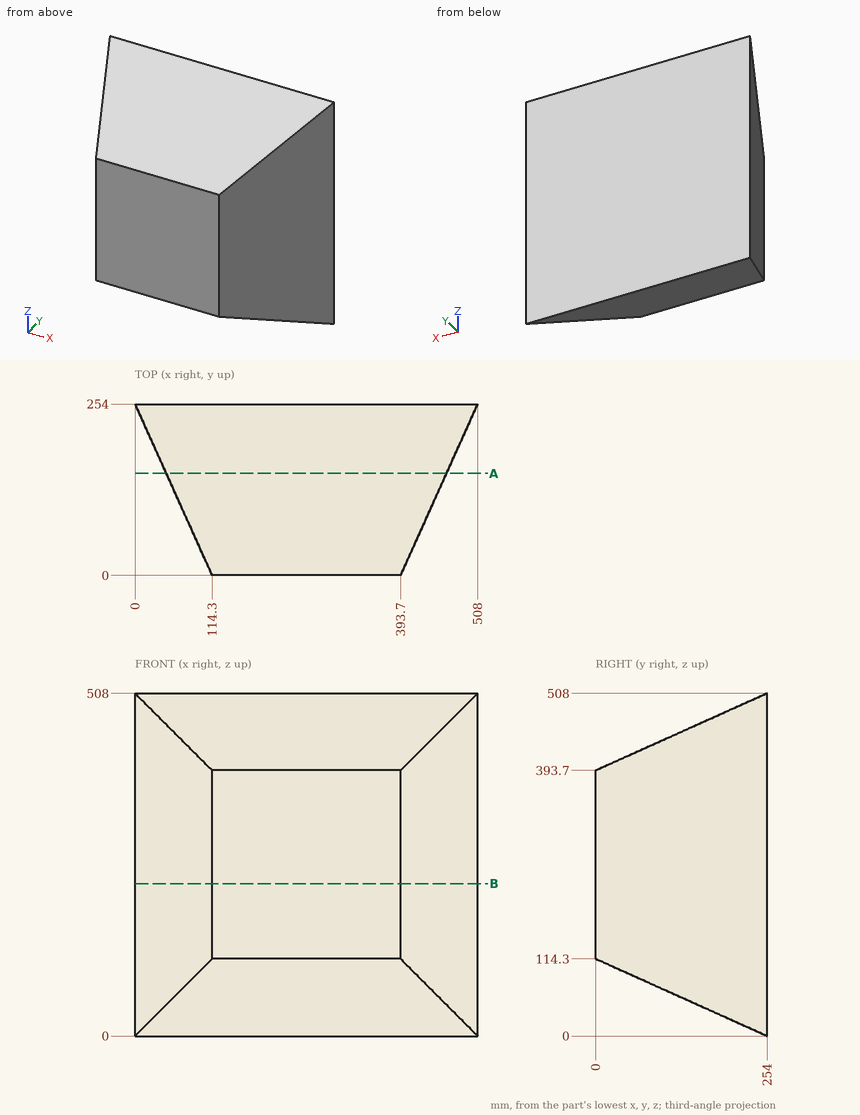
Job drawing, mm, ordinate dimensions from the low corner. One solid piece. Give positions to 0.01 mm unless a question says otherwise; leave off trailing zeros. Order: outer loops, then holes, each group sorted by start corner. A loop starts at its lowest first (then second) coordinate and runs counter-clockwise, first axis right, second up. Notation, with made-up numbers: M 14.5,-25 L 37.5,-25 A20 cw 37.5,-21 Z; hole C -38,54.25 d11. An arc over 180 degrees is marked long. Put each result on its own line as item: value. Start each with the question number.
(1) Drill centre lines: L1, parallel to Z at x = 372, y = 240.5 (3 decimals); L2, parallel to Z at x = 429.5, y = 218; L3, parallel to X at y = 160.5, z = 350 (3 decimals). Where is each one in solid material? Low to high. Write a range as [from, to].
(2) Pin check, flat tips, straight feed: pin 1 Ø10 at (x, y) = (411, 44) entering from +Z; pin 2 Ø6 at (y, z) = (136, 176) entering from -X; pin 3 Ø2 at (x, y) = (238, 201) entering from +Z. Stop position of each tip, or through.
(3) Band-saw the part on A-A on y = 151. Give the cut face in (x, z), then the cut area to 3 significant figures.
(4) Band-saw the part on B-B on z = 226. Give the cut face in (x, y), then the cut area to 4 significant figures.
Results below:
1. L1: z = [6.075, 501.925]
1. L2: z = [16.2, 491.8]
1. L3: x = [42.075, 465.925]
2. pin 1: stops at z = 415.75
2. pin 2: stops at x = 51.75
2. pin 3: stops at z = 484.6
3. outline: M 46.35,46.35 L 461.65,46.35 L 461.65,461.65 L 46.35,461.65 Z
3. area: 172,000 mm2
4. outline: M 0,254 L 114.3,0 L 393.7,0 L 508,254 Z
4. area: 100,000 mm2
